Input: part model. Units: mm. Frame: model coordinates. Give positions to 0.01 mm unless a question says otherwise; leave off trailing zeros. Order: outer loops, then holes, each group sorted by start corner. A loop starts at its lowest first (then second) coordinate and runs counter-clockwise, first axis right, second up. Notation, with made-up numbers: (11.25, 80.5) -> (32.25, 80.5) arc R26 ccw to (32.25, 98.5) -> close; hole circle Ø7 at (46, 36.5). An arc over 180 degrees is marked (long way). Use a Markdown table: item, result. Add a question column.
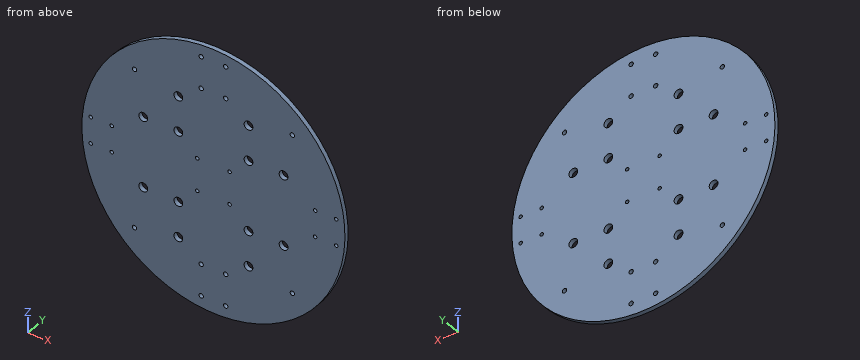
from build123d import *

# Parameters (mm, degrees)
SKETCH_3_R      = 150
SKETCH_3_R_2    = 2
SKETCH_3_R_3    = 2.5
SKETCH_3_R_4    = 5
EXTRUDE_2_DEPTH = 5


with BuildPart() as part:
    # 草图3 → 凸台-拉伸2 (new body)
    with BuildSketch(Plane(origin=(0, 0, 0), x_dir=(1, 0, 0), z_dir=(0, 1, 0))):
        with Locations(Location((0, 0, 0), (0, 0, 270))):
            Circle(SKETCH_3_R)
        with Locations(Location((116, 15, 0), (0, 0, 270))):
            Circle(SKETCH_3_R_2, mode=Mode.SUBTRACT)
        with Locations(Location((140, 15, 0), (0, 0, 270))):
            Circle(SKETCH_3_R_2, mode=Mode.SUBTRACT)
        with Locations(Location((116, -15, 0), (0, 0, 270))):
            Circle(SKETCH_3_R_2, mode=Mode.SUBTRACT)
        with Locations(Location((140, -15, 0), (0, 0, 270))):
            Circle(SKETCH_3_R_2, mode=Mode.SUBTRACT)
        with Locations(Location((-140, -15, 0), (0, 0, 270))):
            Circle(SKETCH_3_R_2, mode=Mode.SUBTRACT)
        with Locations(Location((-140, 15, 0), (0, 0, 270))):
            Circle(SKETCH_3_R_2, mode=Mode.SUBTRACT)
        with Locations(Location((-116, 15, 0), (0, 0, 270))):
            Circle(SKETCH_3_R_2, mode=Mode.SUBTRACT)
        with Locations(Location((-116, -15, 0), (0, 0, 270))):
            Circle(SKETCH_3_R_2, mode=Mode.SUBTRACT)
        with Locations(Location((14, 100, 0), (0, 0, 270))):
            Circle(SKETCH_3_R_3, mode=Mode.SUBTRACT)
        with Locations(Location((-14, 100, 0), (0, 0, 270))):
            Circle(SKETCH_3_R_3, mode=Mode.SUBTRACT)
        with Locations(Location((14, 136, 0), (0, 0, 270))):
            Circle(SKETCH_3_R_3, mode=Mode.SUBTRACT)
        with Locations(Location((-14, 136, 0), (0, 0, 270))):
            Circle(SKETCH_3_R_3, mode=Mode.SUBTRACT)
        with Locations(Location((14, -100, 0), (0, 0, 270))):
            Circle(SKETCH_3_R_3, mode=Mode.SUBTRACT)
        with Locations(Location((14, -136, 0), (0, 0, 270))):
            Circle(SKETCH_3_R_3, mode=Mode.SUBTRACT)
        with Locations(Location((-14, -100, 0), (0, 0, 270))):
            Circle(SKETCH_3_R_3, mode=Mode.SUBTRACT)
        with Locations(Location((-14, -136, 0), (0, 0, 270))):
            Circle(SKETCH_3_R_3, mode=Mode.SUBTRACT)
        with Locations(Location((18.5, 18.5, 0), (0, 0, 270))):
            Circle(SKETCH_3_R_2, mode=Mode.SUBTRACT)
        with Locations(Location((-18.5, 18.5, 0), (0, 0, 270))):
            Circle(SKETCH_3_R_2, mode=Mode.SUBTRACT)
        with Locations(Location((-18.5, -18.5, 0), (0, 0, 270))):
            Circle(SKETCH_3_R_2, mode=Mode.SUBTRACT)
        with Locations(Location((18.5, -18.5, 0), (0, 0, 270))):
            Circle(SKETCH_3_R_2, mode=Mode.SUBTRACT)
        with Locations(Location((90, -90, 0), (0, 0, 270))):
            Circle(SKETCH_3_R_3, mode=Mode.SUBTRACT)
        with Locations(Location((90, 90, 0), (0, 0, 270))):
            Circle(SKETCH_3_R_3, mode=Mode.SUBTRACT)
        with Locations(Location((-90, 90, 0), (0, 0, 270))):
            Circle(SKETCH_3_R_3, mode=Mode.SUBTRACT)
        with Locations(Location((-90, -90, 0), (0, 0, 270))):
            Circle(SKETCH_3_R_3, mode=Mode.SUBTRACT)
        with Locations(Location((40, 40, 0), (0, 0, 270))):
            Circle(SKETCH_3_R_4, mode=Mode.SUBTRACT)
        with Locations(Location((40, -40, 0), (0, 0, 270))):
            Circle(SKETCH_3_R_4, mode=Mode.SUBTRACT)
        with Locations(Location((-40, 40, 0), (0, 0, 270))):
            Circle(SKETCH_3_R_4, mode=Mode.SUBTRACT)
        with Locations(Location((-40, -40, 0), (0, 0, 270))):
            Circle(SKETCH_3_R_4, mode=Mode.SUBTRACT)
        with Locations(Location((80, 40, 0), (0, 0, 270))):
            Circle(SKETCH_3_R_4, mode=Mode.SUBTRACT)
        with Locations(Location((80, -40, 0), (0, 0, 270))):
            Circle(SKETCH_3_R_4, mode=Mode.SUBTRACT)
        with Locations(Location((40, 80, 0), (0, 0, 270))):
            Circle(SKETCH_3_R_4, mode=Mode.SUBTRACT)
        with Locations(Location((-40, 80, 0), (0, 0, 270))):
            Circle(SKETCH_3_R_4, mode=Mode.SUBTRACT)
        with Locations(Location((-80, 40, 0), (0, 0, 270))):
            Circle(SKETCH_3_R_4, mode=Mode.SUBTRACT)
        with Locations(Location((-80, -40, 0), (0, 0, 270))):
            Circle(SKETCH_3_R_4, mode=Mode.SUBTRACT)
        with Locations(Location((-40, -80, 0), (0, 0, 270))):
            Circle(SKETCH_3_R_4, mode=Mode.SUBTRACT)
        with Locations(Location((40, -80, 0), (0, 0, 270))):
            Circle(SKETCH_3_R_4, mode=Mode.SUBTRACT)
    extrude(amount=EXTRUDE_2_DEPTH)


solid = part.part
Q1. Section query C-C (z = 40). Return loops of the section in (x, y).
Q2. Section query D-D (y = 1.9). Give the number of separate pieces and of enclosed holes in the cut face, plus the area to 3 significant figures.
Q3. Ray query, line 1 (X direction, y = 3, z = -18.5); line 2 (Z direction, x = -83.5, y = 1.85); line 3 (X direction, y = 3.35, z = -15). Return the intervals inside material, ascending.
Q4. Section query B-B (x = -40). Return loops of the section in (y, z), plus the area to 3 significant figures.
Q5. First-contact query: pin 1 (1.5 mm diameter, centred on y = 1, z = -47.5, fed in from -X); pin 2 (1 mm diameter, centred on y = 4, z = -28, fed in from -X); pin 3 (3 mm diameter, centred on y = 3.5, z = -103.5, fed in from +X). Flat tips, straight axial feed; report the tip coordinate or a pass-through.
Q6. Section query A-A (x = -80). Return loops of the section in (y, z), plus the area to 3 significant figures.
Solution:
| question | item | result |
|---|---|---|
| 1 | outline | (-144.57, 0) -> (-85, 0) -> (-85, 5) -> (-144.57, 5) -> close; (-75, 0) -> (-45, 0) -> (-45, 5) -> (-75, 5) -> close; (-35, 0) -> (35, 0) -> (35, 5) -> (-35, 5) -> close; (45, 0) -> (75, 0) -> (75, 5) -> (45, 5) -> close; (85, 0) -> (144.57, 0) -> (144.57, 5) -> (85, 5) -> close |
| 2 | separate pieces | 1 |
| 2 | enclosed holes | 36 |
| 2 | area | 69,400 mm² |
| 3 | line 1 | x = -148.85 to -20.5, -16.5 to 16.5, 20.5 to 148.85 |
| 3 | line 2 | z = -124.61 to -43.57, -36.43 to 36.43, 43.57 to 124.61 |
| 3 | line 3 | x = -149.25 to -142, -138 to -118, -114 to 114, 118 to 138, 142 to 149.25 |
| 4 | outline | (0, -144.57) -> (5, -144.57) -> (5, -85) -> (0, -85) -> close; (0, -75) -> (5, -75) -> (5, -45) -> (0, -45) -> close; (0, -35) -> (5, -35) -> (5, 35) -> (0, 35) -> close; (0, 45) -> (5, 45) -> (5, 75) -> (0, 75) -> close; (0, 85) -> (5, 85) -> (5, 144.57) -> (0, 144.57) -> close |
| 4 | area | 1,250 mm² |
| 5 | pin 1 | stops at x = -142.53 |
| 5 | pin 2 | stops at x = -147.46 |
| 5 | pin 3 | stops at x = 109.98 |
| 6 | outline | (0, -126.89) -> (5, -126.89) -> (5, -45) -> (0, -45) -> close; (0, -35) -> (5, -35) -> (5, 35) -> (0, 35) -> close; (0, 45) -> (5, 45) -> (5, 126.89) -> (0, 126.89) -> close |
| 6 | area | 1,170 mm² |
